Read the model definition and answer for the solid it produces. Units are mm, in the model's axes. A direction names the side the tool comes from. Give positions to 0.01 mm unless a question says otherwise; leave off trailing zeros. Order: outer loops, then holes, each group sorted by start corner. A loop starts at its lowest first (then second) coordinate and runs counter-clockwise, first axis right, second up. Notation, with made-up numbers: (39.5, 4) - (52.5, 4) arc R17 cw to (52.5, 25) - close; hole circle Ø1 at (-20.75, -23.75). An arc over 180 degrees is marked (long way). Answer as CSV lines item,"result". Start each with the question number.
from build123d import *

# Parameters (mm, degrees)
F0_W     = 76.200001
F0_H     = 24.130002
F1_DEPTH = 25.4
F2_R     = 8.89
F4_DEPTH = 25.4
F5_R     = 4.445
F6_DEPTH = 25.4


with BuildPart() as f1:
    # F0 (on Top) → F1 (new body)
    with BuildSketch(Plane.XY):
        with Locations((-3.386665, 12.065001)):
            Rectangle(F0_W, F0_H)
    extrude(amount=F1_DEPTH)

    # F2
    f2_edges = [f1.edges().sort_by_distance(p)[0] for p in [
        (-41.486666, 24.130002, 12.7),
        (34.713335, 24.130002, 12.7),
        (-41.486666, 0, 12.7),
        (34.713335, 0, 12.7),
    ]]
    fillet(f2_edges, radius=F2_R)

    # F3 (on face) → F4 (cut)
    with BuildSketch(Plane.XY.offset(25.4)):
        Polygon((25.823335, 24.130002), (-32.596666, 24.130002), (-3.386665, 17.516416), align=None)
        Polygon((25.823335, 0), (-3.386665, 6.613586), (-32.596666, 0), align=None)
    extrude(amount=-F4_DEPTH, mode=Mode.SUBTRACT)

    # F5 (on face) → F6 (join)
    with BuildSketch(Plane(origin=(0, 0, 0), x_dir=(1, 0, 0), z_dir=(0, 0, -1))):
        with BuildLine():
            ThreePointArc((-30.691666, -12.065001), (-35.136666, -7.620001), (-39.581666, -12.065001))
            ThreePointArc((-39.581666, -12.065001), (-35.136666, -16.510001), (-30.691666, -12.065001))
        make_face()
        with Locations((28.363335, -12.065001)):
            Circle(F5_R)
    extrude(amount=F6_DEPTH)


solid = f1.part
(1) Determine the mould class of faces 1 (the flat face through (-4, 12, 25.4)), 2 (the cylindrical face through (32.04, 2.535, 12.878)), 3 (the flat face through (-17.787, 3.353, 12.878)), 4 (the flat face through (11.014, 20.777, 12.878)) for opening direction X: released by +X, released by -X, zero draft, split by the parting line, or undercut.
(2) Section D-D, the plane y = 13 is taken. Write down the section's boundary in (x, z), and give its area (3 significant figures).
(3) Section A-A, the plane y = 5.25 is taken. Write down the section's boundary in (x, z).
(4) Section B-B, the plane z = 2 is taken. Write down the section's boundary in (x, y).
(5) Flat-ended cylindrical pins translate along their axes: pin 1 Ø8 at (x, z) = (-21, 4) entering from -Y; pin 2 Ø5 at (y, z) = (13, -18) entering from +X; pin 3 Ø1 at (x, y) = (20.5, 14.5) entering from -Z. Find the tip coordinate at first contact, or state that the pin passes through.
(6) Section C-C, the plane z = -4.5 is taken. Write down the section's boundary in (x, y) (3 decimals).
(7) Which of the six approach directions +Z, -Z, +X, -X, +Y, -Y give full straight-line access (tool end or side, diameter ignored) to faces 5 (the flat face through (11.42, 3.26, 12.88)), 6 (the cylindrical face through (32.178, 21.457, 12.878)), 7 (the cylindrical face through (-30.696, 12.26, -12.522)), 8 (the flat face through (-18.2, 20.87, 12.88))?
(8) Straight lines are drawn through the part: line 1 (Z direction, x = -10, y = 10.25); line 2 (X direction, y = 9.75, z = -20.5); line 3 (Y direction, x = -8, z = 21). For each, find the intervals that lie inside material, in ascending order. Write a range as [from, to].
Checks:
1,face 1,"zero draft"
1,face 2,"released by +X"
1,face 3,"undercut"
1,face 4,"undercut"
2,outline,"(-41.49, 0) - (-39.48, 0) - (-39.48, -25.4) - (-30.79, -25.4) - (-30.79, 0) - (24.02, 0) - (24.02, -25.4) - (32.71, -25.4) - (32.71, 0) - (34.71, 0) - (34.71, 25.4) - (-41.49, 25.4) - close"
2,area,"2,380 mm²"
3,outline,"(-40.71, 0) - (-9.41, 0) - (-9.41, 25.4) - (-40.71, 25.4) - close; (2.64, 0) - (33.93, 0) - (33.93, 25.4) - (2.64, 25.4) - close"
4,outline,"(-41.49, 8.89) arc R8.89 ccw to (-32.6, 0) - (-3.39, 6.61) - (25.82, 0) arc R8.89 ccw to (34.71, 8.89) - (34.71, 15.24) arc R8.89 ccw to (25.82, 24.13) - (-3.39, 17.52) - (-32.6, 24.13) arc R8.89 ccw to (-41.49, 15.24) - close"
5,pin 1,"stops at y = 1.72"
5,pin 2,"stops at x = 32.81"
5,pin 3,"stops at z = 0"
6,outline,"circle Ø8.89 at (-35.137, 12.065); circle Ø8.89 at (28.363, 12.065)"
7,face 5,"+Z, -Z, -Y"
7,face 6,"+Z, -Z, +X, +Y"
7,face 7,"-Z"
7,face 8,"+Z, -Z, +Y"
8,line 1,"z = [0, 25.4]"
8,line 2,"x = [-38.93, -31.34], [24.57, 32.16]"
8,line 3,"y = [5.57, 18.56]"
